```python
from build123d import *

# Parameters (mm, degrees)
AUFSATZ_LINEAR_AUSTRAGEN1_DEPTH = 4
SKIZZE2_R                       = 3.05
AUFSATZ_LINEAR_AUSTRAGEN2_DEPTH = 18.5
AUFSATZ_LINEAR_START            = 15.5
AUFSATZ_LINEAR_AUSTRAGEN3_DEPTH = 1.6
SCHNITT_LINEAR_AUSTRAGEN1_REACH = 25.766
SKIZZE4_R                       = 1.3
FASE1_SIZE                      = 0.4


with BuildPart() as part:
    # Skizze1 → Aufsatz-Linear austragen1 (new body)
    with BuildSketch(Plane.XY):
        with BuildLine():
            Line((-4, 4.472135955), (-4, -4.472135955))
            ThreePointArc((-4, -4.472135955), (0, -6), (4, -4.472135955))
            Line((4, -4.472135955), (4, 4.472135955))
            ThreePointArc((4, 4.472135955), (0, 6), (-4, 4.472135955))
        make_face()
    extrude(amount=AUFSATZ_LINEAR_AUSTRAGEN1_DEPTH)

    # Skizze2 → Aufsatz-Linear austragen2 (add)
    with BuildSketch(Plane.XY.offset(4)):
        Circle(SKIZZE2_R)
    extrude(amount=AUFSATZ_LINEAR_AUSTRAGEN2_DEPTH)

    # Skizze3 → Aufsatz-Linear austragen3 (add)
    with BuildSketch(Plane.XY.offset(4).offset(AUFSATZ_LINEAR_START)):
        with BuildLine():
            Line((3.5, 1.25), (2.782085549, 1.25))
            ThreePointArc((2.782085549, 1.25), (2.982269348, 0.639194445), (3.05, 0))
            ThreePointArc((3.05, 0), (2.982269348, -0.639194445), (2.782085549, -1.25))
            Line((2.782085549, -1.25), (3.5, -1.25))
            ThreePointArc((3.5, -1.25), (4.75, 0), (3.5, 1.25))
        make_face()
    extrude(amount=AUFSATZ_LINEAR_AUSTRAGEN3_DEPTH)

    # Skizze4 → Schnitt-Linear austragen1 (cut, up to next)
    with BuildSketch(Plane.XY.offset(22.5), mode=Mode.PRIVATE) as schnitt_linear_austragen1_sk1:
        Circle(SKIZZE4_R)
    schnitt_linear_austragen1_tool1 = extrude(schnitt_linear_austragen1_sk1.sketch, amount=-SCHNITT_LINEAR_AUSTRAGEN1_REACH, mode=Mode.PRIVATE) & part.part
    add(schnitt_linear_austragen1_tool1.solids().sort_by_distance((0, 0, 22.5))[0], mode=Mode.SUBTRACT)

    # Fase1
    fase1_edges = [part.edges().sort_by_distance(p)[0] for p in [
        (-3.05, 0, 22.5),
    ]]
    chamfer(fase1_edges, length=FASE1_SIZE)


solid = part.part
```
Source: CAD feature listing. Evaluate the final solid. Frame: model axes, mm. A direction names the side the tool comes from. Coordinates: 2 decimals unless noted, no trailing zeros. Loops run counter-clockwise (first coordinate to the right, second up) from the corner with the lowest first, then second, coordinate; pieces in that order, holes last. Notation, with made-up numbers: (-18.5, -24) - (7.5, -24) arc R20 ccw to (7.5, -2) - close; hole circle Ø6 at (70, 33.5). An arc over 180 degrees is marked (long way). Answer as CSV lines item,"result".
1. Contact query for flat-ended pins moving along their axis: pin 1 (1.6 mm diameter, centred on x = 3.5, y = -0.5, fed in from +Z); pin 2 (0.8 mm diameter, centred on x = 3, z = 20.5, fed in from -Y); pin 3 (1 mm diameter, centred on y = 2, z = 11.5, fed in from +X). Output: stop coordinate, or through.
Established:
pin 1,"stops at z = 22.41"
pin 2,"stops at y = -1.59"
pin 3,"stops at x = 2.66"
2. Section A-A (x = 0). Return loops of the section in (y, z).
Established:
outline,"(-6, 0) - (-1.3, 0) - (-1.3, 22.5) - (-2.65, 22.5) - (-3.05, 22.1) - (-3.05, 4) - (-6, 4) - close; (1.3, 0) - (6, 0) - (6, 4) - (3.05, 4) - (3.05, 22.1) - (2.65, 22.5) - (1.3, 22.5) - close"
3. Section B-B (y = 0). Return loops of the section in (x, z).
Established:
outline,"(-4, 0) - (-1.3, 0) - (-1.3, 22.5) - (-2.65, 22.5) - (-3.05, 22.1) - (-3.05, 4) - (-4, 4) - close; (1.3, 0) - (4, 0) - (4, 4) - (3.05, 4) - (3.05, 19.5) - (4.75, 19.5) - (4.75, 21.1) - (3.05, 21.1) - (3.05, 22.1) - (2.65, 22.5) - (1.3, 22.5) - close"
4. Mould query, pull axis X, two halves, no side actions, for faces 6 (the cylindrical face through (0, -6, 2)), 7 (the cylindrical face through (-0.17, 1.29, 11.41)), 8 (the flat face through (0.83, -1.25, 0)). Classes: released by +X, released by -X, zero draft, split by the parting line, or undercut.
Established:
face 6,"split by the parting line"
face 7,"undercut"
face 8,"zero draft"
5. Ray query, line 1 (Y direction, x = 0, z = 14); line 2 (Z direction, x = 0, y = -3.5); line 3 (Y direction, x = 1.5, z = 21.25). Return the intervals inside material, ascending.
Established:
line 1,"y = -3.05 to -1.3, 1.3 to 3.05"
line 2,"z = 0 to 4"
line 3,"y = -2.66 to 2.66"
6. Section D-D (y = 4). Return loops of the section in (x, z), then the cut area to 3 significant figures.
Established:
outline,"(-4, 0) - (4, 0) - (4, 4) - (-4, 4) - close"
area,"32.0 mm2"
7. Reachability of faces 1 (the cylindrical face through (-3.047, 0.134, 12.923)), 2 (the flat face through (-4, 0, 2)), 3 (the cylindrical face through (4.75, -0.03, 20.29)), 4 (the flat face through (4, 0, 2)), 5 (the cylindrical face through (0, 6, 2)) from +Z, -Z, +X, -X, +Y, -Y: full face, straight path, thin tool, end or side. Return the list, or none.
Established:
face 1,"none"
face 2,"+Z, -Z, -X, +Y, -Y"
face 3,"+Z, +X"
face 4,"-Z, +X, +Y, -Y"
face 5,"+Z, -Z, +Y"
8. Section C-C (z = 19.25). Return loops of the section in (x, y), then the cut area to 3 significant figures.
Established:
outline,"circle Ø6.1 at (0, 0); hole circle Ø2.6 at (0, 0)"
area,"23.9 mm2"
